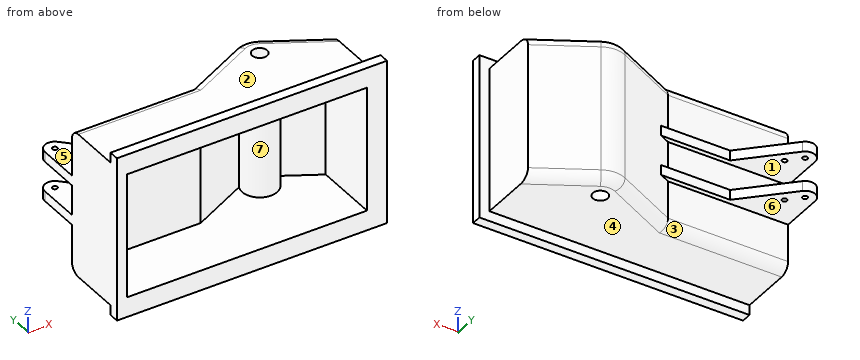
```python
from build123d import *

# Parameters (mm, degrees)
SKETCH1_R           = 15
BOSS_EXTRUDE1_DEPTH = 145
BOSS_EXTRUDE2_START = 30
SKETCH2_R           = 5
BOSS_EXTRUDE2_DEPTH = 20
SHELL1_START        = -125
SHELL1_DEPTH        = 250
SKETCH3_W           = 520
SKETCH3_H           = 290
BOSS_EXTRUDE3_DEPTH = 20
FILLET1_R           = 20


# Read off the part's stored shape, not the designer's step: Shell1
with BuildPart() as part:
    # Sketch1 → Boss-Extrude1 (new, symmetric)
    with BuildSketch(Plane.XY):
        with BuildLine():
            Line((-260, 0), (260, 0))
            Line((260, 0), (260, 120))
            Line((260, 120), (153.093568272, 180.972007347))
            ThreePointArc((153.093568272, 180.972007347), (129.803653925, 187.517381697), (106.167012988, 182.362651739))
            Line((106.167012988, 182.362651739), (-20, 120))
            Line((-20, 120), (-260, 120))
            Line((-260, 120), (-260, 0))
        make_face()
        with Locations((128.322579774, 140)):
            Circle(SKETCH1_R, mode=Mode.SUBTRACT)
    extrude(amount=BOSS_EXTRUDE1_DEPTH, both=True)

    # Sketch2 → Boss-Extrude2 (add)
    with BuildSketch(Plane.XY.offset(BOSS_EXTRUDE2_START)):
        with BuildLine():
            Line((-260, 120), (-260, 204))
            ThreePointArc((-260, 204), (-247.653668647, 222.47759065), (-225.857864376, 218.142135624))
            Line((-225.857864376, 218.142135624), (-137.715728753, 130))
            Line((-137.715728753, 130), (0.23118156, 130))
            Line((0.23118156, 130), (-20, 120))
            Line((-20, 120), (-260, 120))
        make_face()
        with Locations((-240, 204)):
            Circle(SKETCH2_R, mode=Mode.SUBTRACT)
        with Locations((-215, 179)):
            Circle(SKETCH2_R, mode=Mode.SUBTRACT)
    boss_extrude2 = extrude(amount=BOSS_EXTRUDE2_DEPTH)

    # Mirror1: Boss-Extrude2 across plane
    add(boss_extrude2.mirror(Plane.XY))

    # Shell1 outline → Shell1 (cut)
    with BuildSketch(Plane.XY.offset(SHELL1_START)):
        with BuildLine():
            Line((96.937260838, 155.490698991), (-15.32697978, 100))
            Line((-15.32697978, 100), (-240, 100))
            Line((-240, 100), (-240, 0))
            Line((-240, 0), (240, 0))
            Line((240, 0), (240, 108.382476706))
            Line((240, 108.382476706), (160.526102167, 153.708871052))
            ThreePointArc((160.526102167, 153.708871052), (127.342226815, 105.013732579), (96.937260838, 155.490698991))
        make_face()
    extrude(amount=SHELL1_DEPTH, mode=Mode.SUBTRACT)

    # Sketch3 → Boss-Extrude3 (add)
    # profile 1 of 2: a face of its own
    with BuildSketch(Plane.XZ):
        Rectangle(SKETCH3_W, SKETCH3_H)
        Polygon((160.526102167, -125), (-240, -125), (-240, 125), (-15.32697978, 125), (93.322579774, 125), (96.937260838, 125), (163.322579774, 125), (240, 125), (240, -125), align=None, mode=Mode.SUBTRACT)
    # profile 2 of 2: a face of its own
    with BuildSketch(Plane.XZ):
        Polygon((280, 165), (-260, 165), (-260, 145), (260, 145), (260, -145), (-260, -145), (-260, -165), (280, -165), align=None)
    extrude(amount=BOSS_EXTRUDE3_DEPTH)

    # Fillet1
    fillet1_edges = [part.edges().sort_by_distance(p)[0] for p in [
        (129.803653925, 187.517381697, -145),
        (-140, 120, 145),
        (206.546784136, 150.486003673, 145),
        (129.803653925, 187.517381697, 145),
        (206.546784136, 150.486003673, -145),
        (43.083506494, 151.181325869, 145),
        (-140, 120, -145),
        (43.083506494, 151.181325869, -145),
    ]]
    fillet(fillet1_edges, radius=FILLET1_R)


solid = part.part
```
Check sheet for the modelled part. Datum: model origin and axes. Units: mm. Face numbers are marked on the shaded views. A direction names the side the tool comes from. Give positions to 0.01 mm unless a question says otherwise; leave off trailing zeros. Write each loop counter-clockwise with the first axis right and the second up, starting at its lowest first coordinate (ties: lowest second). Pieces come first, ordered by that corner, then holes. Notation, with made-up numbers: (-23, -5.5) - (30, -5.5) arc R12 cw to (30, -0.5) - close; hole circle Ø11 at (73, 77). An arc over 180 degrees is marked (long way). Answer as a JSON object with one key per item and string values. Group by question number.
1) Sectioned sample at A-A (z = 83). Record the cut outline in (x, y).
2) Sectioned sample at D-D (z = -134). Record the cut outline in (x, y), then the cut area to 3 significant figures.
3) Release check for a two-part mould opening along Z. For the marked faces 1, 2 and 3 record: pulls with the +Z half, pulls with the -Z half, needs draft (parallel to the pull), parting line crosses it, or undercut.
4) Sectioned sample at C-C (x = -25.5). Record the cut outline in (y, z), then the cut area to 3 significant figures.
5) Access from +Z, -Z, +X, -X, +Y, -Y to the whole of each face (thin tool, end or side, straight path). Record for the marked faces 4, 5, 6 and 7.
6) Sectioned sample at B-B (y = 67.5). Record the cut outline in (x, z), then the cut area to 3 significant figures.
7) Thickness scan on probe 1 along Z at (x, y) = (-195, 13); probe 2 along X at (y, z) = (91, 52.5); probe 3 along Y at (x, z) = (-215, 35). Record the ranges inside material, lowest first. Write a range as from..to.
8) Depth check by flat-ended pin: P1, Ø4, axis at x = -63, y = 122.5, coming from the +Z side; P2, Ø6, axis at x = -93, y = 81, coming from the +Z side; P3, Ø2, axis at x = -106.5, y = 55, coming from the -Z side. Enter the tip coordinate at first touch or a pass-through.
Geometry results:
{
 "1": {"outline": "(-260, -20) - (-240, -20) - (-240, 100) - (-15.33, 100) - (96.94, 155.49) arc R35 ccw (long way) to (160.53, 153.71) - (240, 108.38) - (240, -20) - (280, -20) - (280, 0) - (260, 0) - (260, 120) - (153.09, 180.97) arc R50 ccw to (106.17, 182.36) - (-20, 120) - (-260, 120) - close; hole circle Ø30 at (128.32, 140)"},
 "2": {"outline": "(-260, -20) - (280, -20) - (280, 0) - (260, 0) - (260, 117.54) - (152.03, 179.11) arc R47.86 ccw to (107.12, 180.44) - (-19.5, 117.86) - (-260, 117.86) - close; hole circle Ø30 at (128.32, 140)", "area": "81,600 mm^2"},
 "3": {"face 1": "undercut", "face 2": "pulls with the +Z half", "face 3": "pulls with the -Z half"},
 "4": {"outline": "(-20, -165) - (0, -165) - (0, -145) - (100, -145) arc R20 ccw to (120, -125) - (120, -50) - (130, -50) - (130, -30) - (120, -30) - (120, 30) - (130, 30) - (130, 50) - (120, 50) - (120, 125) arc R20 ccw to (100, 145) - (0, 145) - (0, 165) - (-20, 165) - (-20, 125) - (100, 125) - (100, -125) - (-20, -125) - close", "area": "11,600 mm^2"},
 "5": {"face 4": "-Z, +X, -X, +Y", "face 5": "+Z, -X, +Y", "face 6": "-Z, -X, +Y", "face 7": "none"},
 "6": {"outline": "(-260, -145) - (260, -145) - (260, 145) - (-260, 145) - close; hole (-240, -125) - (240, -125) - (240, 125) - (-240, 125) - close", "area": "30,800 mm^2"},
 "7": {"probe 1": "z = -145..-125, 125..145", "probe 2": "x = -260..-240, 240..260", "probe 3": "y = 100..174, 184..207.28"},
 "8": {"P1": "stops at z = 50", "P2": "stops at z = 145", "P3": "stops at z = -145"}
}
